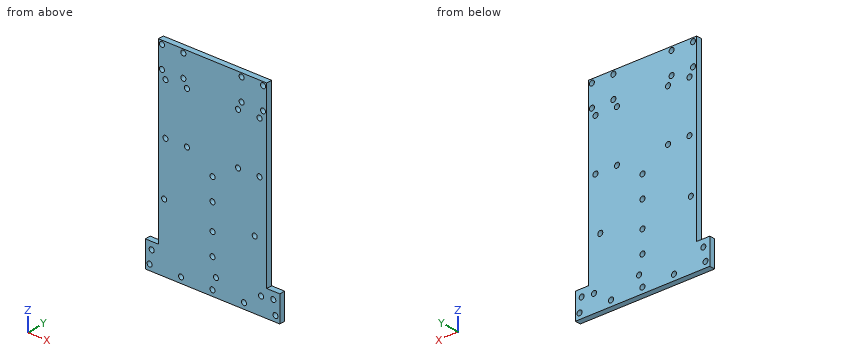
```python
from build123d import *

# Parameters (mm, degrees)
SKETCH1_W           = 75.7
SKETCH1_H           = 42.7
SKETCH1_R           = 1.75
BOSS_EXTRUDE1_DEPTH = 4
SKETCH3_W           = 75.7
SKETCH3_H           = 29.75
SKETCH3_R           = 1.75
BOSS_EXTRUDE2_DEPTH = 4
SKETCH3_3_R         = 1.75
CUT_EXTRUDE1_DEPTH  = 4
SKETCH4_W           = 75.7
SKETCH4_H           = 40
SKETCH4_R           = 1.75
BOSS_EXTRUDE3_DEPTH = 4
BOSS_EXTRUDE4_DEPTH = 4
SKETCH6_3_R         = 1.75
CUT_EXTRUDE2_DEPTH  = 103.587572347
SKETCH7_W           = 9.15
SKETCH7_H           = 10
SKETCH7_R           = 1.75
BOSS_EXTRUDE5_DEPTH = 4
SKETCH8_W           = 75.7
SKETCH8_H           = 20.2
BOSS_EXTRUDE6_DEPTH = 4
SKETCH9_R           = 1.75
CUT_EXTRUDE3_DEPTH  = 121.882959924


with BuildPart() as part:
    # Sketch1 → Boss-Extrude1 (new body)
    with BuildSketch(Plane(origin=(0, 0, 0), x_dir=(1, 0, 0), z_dir=(0, 1, 0))):
        Rectangle(SKETCH1_W, SKETCH1_H)
        with Locations(Location((2.4, 17.25, 0), (0, 0, 270))):
            Circle(SKETCH1_R, mode=Mode.SUBTRACT)
        with Locations(Location((-33.8, -17.05, 0), (0, 0, 270))):
            Circle(SKETCH1_R, mode=Mode.SUBTRACT)
        with Locations(Location((29.5, -17.05, 0), (0, 0, 270))):
            Circle(SKETCH1_R, mode=Mode.SUBTRACT)
        with Locations(Location((33.9, 17.25, 0), (0, 0, 270))):
            Circle(SKETCH1_R, mode=Mode.SUBTRACT)
    extrude(amount=BOSS_EXTRUDE1_DEPTH)

    # Sketch3 → Boss-Extrude2 (add)
    with BuildSketch(Plane(origin=(0, 4, 0), x_dir=(1, 0, 0), z_dir=(0, 1, 0))):
        with Locations((0, -36.225)):
            Rectangle(SKETCH3_W, SKETCH3_H)
        with Locations(Location((0, -42.2, 0), (0, 0, 270))):
            Circle(SKETCH3_R, mode=Mode.SUBTRACT)
        with Locations(Location((0, -27.2, 0), (0, 0, 270))):
            Circle(SKETCH3_R, mode=Mode.SUBTRACT)
    extrude(amount=-BOSS_EXTRUDE2_DEPTH)

    # Sketch3_3 → Cut-Extrude1 (cut)
    with BuildSketch(Plane(origin=(0, 4, 0), x_dir=(1, 0, 0), z_dir=(0, 1, 0))):
        with Locations(Location((0, 5.6, 0), (0, 0, 270))):
            Circle(SKETCH3_3_R)
        with Locations(Location((0, -9.4, 0), (0, 0, 270))):
            Circle(SKETCH3_3_R)
    extrude(amount=-CUT_EXTRUDE1_DEPTH, mode=Mode.SUBTRACT)

    # Sketch4 → Boss-Extrude3 (add)
    # profile 1 of 2: a face of its own
    with BuildSketch(Plane(origin=(0, 0, 0), x_dir=(1, 0, 0), z_dir=(0, 1, 0))):
        with Locations((0, -71.1)):
            Rectangle(SKETCH4_W, SKETCH4_H)
        with Locations(Location((-32.85, -53.6, 0), (0, 0, 270))):
            Circle(SKETCH4_R, mode=Mode.SUBTRACT)
        with Locations(Location((-17.85, -53.6, 0), (0, 0, 270))):
            Circle(SKETCH4_R, mode=Mode.SUBTRACT)
        with Locations(Location((-17.85, -88.6, 0), (0, 0, 270))):
            Circle(SKETCH4_R, mode=Mode.SUBTRACT)
        with Locations(Location((-32.85, -88.6, 0), (0, 0, 270))):
            Circle(SKETCH4_R, mode=Mode.SUBTRACT)
        with Locations(Location((32.85, -88.6, 0), (0, 0, 90))):
            Circle(SKETCH4_R, mode=Mode.SUBTRACT)
        with Locations(Location((17.85, -88.6, 0), (0, 0, 90))):
            Circle(SKETCH4_R, mode=Mode.SUBTRACT)
        with Locations(Location((17.85, -53.6, 0), (0, 0, 90))):
            Circle(SKETCH4_R, mode=Mode.SUBTRACT)
        with Locations(Location((32.85, -53.6, 0), (0, 0, 90))):
            Circle(SKETCH4_R, mode=Mode.SUBTRACT)
    # profile 2 of 2: a face of its own
    with BuildSketch(Plane(origin=(0, 0, 0), x_dir=(1, 0, 0), z_dir=(0, 1, 0))):
        Polygon((-37.85, 21.35), (-44, 21.35), (-44, 29.35), (44, 29.35), (44, 21.35), (37.85, 21.35), align=None)
    extrude(amount=BOSS_EXTRUDE3_DEPTH)

    # Sketch6 → Boss-Extrude4 (add)
    with BuildSketch(Plane(origin=(0, 4, 0), x_dir=(1, 0, 0), z_dir=(0, 1, 0))):
        with BuildLine():
            Line((-44, 27.1), (-44, 29.35))
            Line((-44, 29.35), (-47, 29.35))
            Line((-47, 29.35), (-47, 21.35))
            Line((-47, 21.35), (-44, 21.35))
            Line((-44, 21.35), (-44, 23.6))
            ThreePointArc((-44, 23.6), (-45.75, 25.35), (-44, 27.1))
        make_face()
        with BuildLine():
            Line((47, 29.35), (44, 29.35))
            Line((44, 29.35), (44, 27.1))
            ThreePointArc((44, 27.1), (45.75, 25.35), (44, 23.6))
            Line((44, 23.6), (44, 21.35))
            Line((44, 21.35), (47, 21.35))
            Line((47, 21.35), (47, 29.35))
        make_face()
    extrude(amount=-BOSS_EXTRUDE4_DEPTH)

    # Sketch6_3 → Cut-Extrude2 (cut, through all)
    with BuildSketch(Plane(origin=(0, 4, 0), x_dir=(1, 0, 0), z_dir=(0, 1, 0))):
        with Locations(Location((0, 25.35, 0), (0, 0, 270))):
            Circle(SKETCH6_3_R)
        with Locations(Location((22, 25.35, 0), (0, 0, 270))):
            Circle(SKETCH6_3_R)
        with Locations(Location((44, 25.35, 0), (0, 0, 270))):
            Circle(SKETCH6_3_R)
        with Locations(Location((-22, 25.35, 0), (0, 0, 270))):
            Circle(SKETCH6_3_R)
        with Locations(Location((-44, 25.35, 0), (0, 0, 270))):
            Circle(SKETCH6_3_R)
    extrude(amount=-CUT_EXTRUDE2_DEPTH, mode=Mode.SUBTRACT)

    # Sketch7 → Boss-Extrude5 (add)
    # profile 1 of 2: a face of its own
    with BuildSketch(Plane(origin=(0, 0, 0), x_dir=(1, 0, 0), z_dir=(0, 1, 0))):
        with Locations((-42.425, 16.35)):
            Rectangle(SKETCH7_W, SKETCH7_H)
        with Locations(Location((-42.5, 16.35, 0), (0, 0, 270))):
            Circle(SKETCH7_R, mode=Mode.SUBTRACT)
    # profile 2 of 2: a face of its own
    with BuildSketch(Plane(origin=(0, 0, 0), x_dir=(1, 0, 0), z_dir=(0, 1, 0))):
        with Locations((42.425, 16.35)):
            Rectangle(SKETCH7_W, SKETCH7_H)
        with Locations(Location((42.5, 16.35, 0), (0, 0, 270))):
            Circle(SKETCH7_R, mode=Mode.SUBTRACT)
    extrude(amount=BOSS_EXTRUDE5_DEPTH)

    # Sketch8 → Boss-Extrude6 (add)
    with BuildSketch(Plane(origin=(0, 0, 0), x_dir=(1, 0, 0), z_dir=(0, 1, 0))):
        with Locations((0, -101.2)):
            Rectangle(SKETCH8_W, SKETCH8_H)
    extrude(amount=BOSS_EXTRUDE6_DEPTH)

    # Sketch9 → Cut-Extrude3 (cut, through all)
    with BuildSketch(Plane(origin=(0, 4, 0), x_dir=(1, 0, 0), z_dir=(0, 1, 0))):
        with Locations(Location((-35.35, -93.8, 0), (0, 0, 270))):
            Circle(SKETCH9_R)
        with Locations(Location((-20.35, -93.8, 0), (0, 0, 270))):
            Circle(SKETCH9_R)
        with Locations(Location((-20.35, -108.8, 0), (0, 0, 270))):
            Circle(SKETCH9_R)
        with Locations(Location((-35.35, -108.8, 0), (0, 0, 270))):
            Circle(SKETCH9_R)
    cut_extrude3 = extrude(amount=-CUT_EXTRUDE3_DEPTH, mode=Mode.SUBTRACT)

    # Mirror1: Cut-Extrude3 across plane
    add(cut_extrude3.mirror(Plane(origin=(0, 0, 0), x_dir=(0, 0, 1), z_dir=(1, 0, 0))), mode=Mode.SUBTRACT)


solid = part.part
```
Geometry: final body of the model. Coordinates: model frame, mm. Coordinates: 2 decimals unless noted, no trailing zeros. Order: outer loops, then holes, each group sorted by start corner. A loop starts at its lowest first (then second) coordinate and runs counter-clockwise, first axis right, second up. Notation, with made-up numbers: M 37.5,43 L 73.5,43 A19 ccw 73.5,80 Z; hole C 36.5,38 d6. An arc over 180 degrees is marked long. Answer as CSV lines item,"result".
Q1. Section A-A on z = 93.8. Return the cut outline in (x, y).
Answers:
outline,"M -37.85,0 L -37.1,0 L -37.1,4 L -37.85,4 Z; M -33.6,0 L -22.1,0 L -22.1,4 L -33.6,4 Z; M -18.6,0 L 18.6,0 L 18.6,4 L -18.6,4 Z; M 22.1,0 L 33.6,0 L 33.6,4 L 22.1,4 Z; M 37.1,0 L 37.85,0 L 37.85,4 L 37.1,4 Z"
Q2. Section C-C on y = 0.85. Count the separate pieces of the cut face and the enclosed holes in it, and give its area (3 significant figures).
Answers:
separate pieces,"1"
enclosed holes,"31"
area,"10,700 mm^2"
Q3. First-contact query: P1, Ø1.5, axis at x = 12, z = 83, coming from the -Y side; P2, Ø1.2, axis at y = 2.5, z = 64.5, coming from the -X side. Flat tips, straight axial feed; report the tip coordinate or a pass-through.
Answers:
P1,"stops at y = 0"
P2,"stops at x = -37.85"
Q4. Line query: probe 1 along X at (y, z) = (1.35, 53.6); probe 2 along X at (y, z) = (3.2, 108.8); probe 3 along Z at (x, y) = (-20, 1.3). Output: solid intervals per line, ascending. Write a range as [from, to].
Answers:
probe 1,"x = [-37.85, -34.6], [-31.1, -19.6], [-16.1, 16.1], [19.6, 31.1], [34.6, 37.85]"
probe 2,"x = [-37.85, -37.1], [-33.6, -22.1], [-18.6, 18.6], [22.1, 33.6], [37.1, 37.85]"
probe 3,"z = [-29.35, 92.09], [95.51, 107.09], [110.51, 111.3]"
Q5. Section B-B on z = 27.2. Return the cut outline in (x, y).
Answers:
outline,"M -37.85,0 L -1.75,0 L -1.75,4 L -37.85,4 Z; M 1.75,0 L 37.85,0 L 37.85,4 L 1.75,4 Z"
